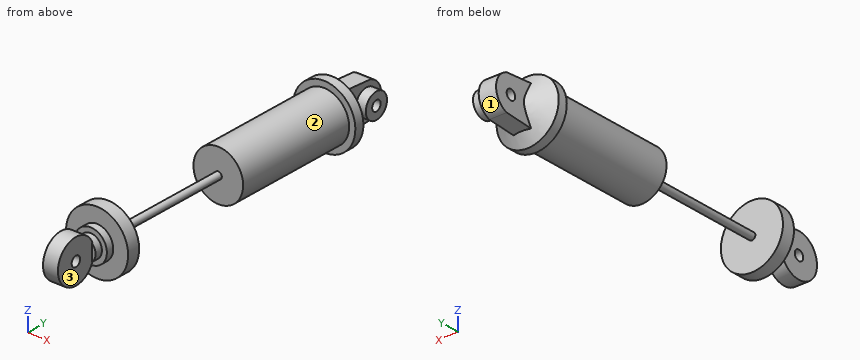
from build123d import *

# Parameters (mm, degrees)
SKETCH1_R      = 7.9375
EXTRUDE1_DEPTH = 70.485
SKETCH4_R      = 1.27
EXTRUDE2_DEPTH = 2.2225
SKETCH5_R      = 5.3975
SKETCH5_R_2    = 1.27
EXTRUDE3_DEPTH = 1.905
SKETCH6_R      = 4.1275
EXTRUDE4_DEPTH = 1.905
SKETCH7_R      = 2.8575
EXTRUDE5_DEPTH = 1.905
SKETCH8_R      = 3.175
SKETCH8_R_2    = 1.27
EXTRUDE6_DEPTH = 2.54
SKETCH9_R      = 7.9375
SKETCH9_R_2    = 6.35
EXTRUDE7_DEPTH = 33.02
SKETCH10_R     = 8.451029387
SKETCH10_R_2   = 0.889
EXTRUDE8_DEPTH = 33.02


with BuildPart() as part:
    # Sketch1 → Extrude1 (new body)
    with BuildSketch(Plane(origin=(0, 0, 0), x_dir=(1, 0, 0), z_dir=(0, 1, 0))):
        with Locations(Location((0, 0, 0), (0, 0, 270))):
            Circle(SKETCH1_R)
    extrude(amount=-EXTRUDE1_DEPTH)

    # Loft1: read off the stored shape, not the designer's step
    # Loft1: loft between two sections, ruled curve by curve
    loft1_from = [
        Edge.make_bspline([(3.207196431, 0, 7.26070226), (17.72860095, 0, 0.846309398), (11.314208088, 0, -13.675095122), (-3.207196431, 0, -7.26070226), (-17.72860095, 0, -0.846309398), (-11.314208088, 0, 13.675095122), (3.207196431, 0, 7.26070226)], [0, 0, 0, 0, 0.5, 0.5, 0.5, 1, 1, 1, 1], 3, [1, 0.333333333, 0.333333333, 1, 0.333333333, 0.333333333, 1]),
    ]
    loft1_to = [
        Edge.make_bspline([(0.075387957, 3.937, 1.903507724), (3.882403406, 3.937, 1.75273181), (3.731627491, 3.937, -2.054283639), (-0.075387957, 3.937, -1.903507724), (-3.882403406, 3.937, -1.75273181), (-3.731627491, 3.937, 2.054283639), (0.075387957, 3.937, 1.903507724)], [0, 0, 0, 0, 0.5, 0.5, 0.5, 1, 1, 1, 1], 3, [1, 0.333333333, 0.333333333, 1, 0.333333333, 0.333333333, 1]),
    ]
    loft1 = Solid(Shell([*[Face.make_surface_from_curves(loft1_from[k], loft1_to[k]) for k in range(1)], Face(Wire(loft1_from)), Face(Wire(loft1_to))]))
    add(loft1)

    # Sketch4 → Extrude2 (add, symmetric)
    with BuildSketch(Plane(origin=(0, 0, 0), x_dir=(0, 0, -1), z_dir=(1, 0, 0))):
        with BuildLine():
            Line((4.965601833, 1.905), (4.445, 8.89))
            ThreePointArc((4.445, 8.89), (0, 12.065), (-4.445, 8.89))
            Line((-4.445, 8.89), (-4.965601949, 1.905))
            Line((-4.965601949, 1.905), (-5.107584298, 0))
            Line((-5.107584298, 0), (5.107584151, 0))
            Line((5.107584151, 0), (4.965601833, 1.905))
        make_face()
        with Locations((0, 7.62)):
            Circle(SKETCH4_R, mode=Mode.SUBTRACT)
    extrude(amount=EXTRUDE2_DEPTH, both=True)

    # Sketch6 → Extrude4 (add)
    with BuildSketch(Plane.XZ.offset(70.485)):
        with Locations(Location((0, 0, 0), (0, 0, 90))):
            Circle(SKETCH6_R)
    extrude(amount=EXTRUDE4_DEPTH)



with BuildPart() as body_2:
    # Sketch5 → Extrude3 (new, symmetric)
    with BuildSketch(Plane(origin=(0, 0, 0), x_dir=(0, 0, -1), z_dir=(1, 0, 0))):
        with Locations(Location((0, -79.0575, 0), (0, 0, 180))):
            Circle(SKETCH5_R)
        with Locations(Location((0, -79.0575, 0), (0, 0, 180))):
            Circle(SKETCH5_R_2, mode=Mode.SUBTRACT)
    extrude(amount=EXTRUDE3_DEPTH, both=True)


with BuildPart() as part_1:
    add(part.part)

    add(body_2.part)  # Extrude5 merges body 2
    # Sketch7 → Extrude5 (add)
    with BuildSketch(Plane.XZ.offset(72.39)):
        with Locations(Location((0, 0, 0), (0, 0, 117.266044451))):
            Circle(SKETCH7_R)
    extrude(amount=EXTRUDE5_DEPTH)

    # Sketch8 → Extrude6 (add)
    with BuildSketch(Plane(origin=(2.2225, 0, 0), x_dir=(0, 0, -1), z_dir=(1, 0, 0))):
        with Locations(Location((0, 7.62, 0), (0, 0, 180))):
            Circle(SKETCH8_R)
        with Locations((0, 7.62)):
            Circle(SKETCH8_R_2, mode=Mode.SUBTRACT)
    extrude(amount=EXTRUDE6_DEPTH)

    # Sketch9 → Extrude7 (cut)
    with BuildSketch(Plane(origin=(0, -2.413, 0), x_dir=(-1, 0, 0), z_dir=(0, 1, 0))):
        with Locations(Location((0, 0, 0), (0, 0, 90))):
            Circle(SKETCH9_R)
        with Locations(Location((0, 0, 0), (0, 0, 90))):
            Circle(SKETCH9_R_2, mode=Mode.SUBTRACT)
    extrude(amount=-EXTRUDE7_DEPTH, mode=Mode.SUBTRACT)

    # Sketch10 → Extrude8 (cut)
    with BuildSketch(Plane(origin=(0, -34.163, 0), x_dir=(-1, 0, 0), z_dir=(0, 1, 0))):
        Circle(SKETCH10_R)
        with Locations(Location((0, 0, 0), (0, 0, 90))):
            Circle(SKETCH10_R_2, mode=Mode.SUBTRACT)
    extrude(amount=-EXTRUDE8_DEPTH, mode=Mode.SUBTRACT)


solid = part_1.part
Check sheet for the modelled part. Datum: model origin and axes. Units: mm. Face numbers are marked on the shaded views. Give positions to 0.01 mm unless a question says otherwise; leave off trailing zeros. Order: outer loops, then holes, each group sorted by start corner. A loop starts at its lowest first (then second) coordinate and runs counter-clockwise, first axis right, second up. Notation, with made-up numbers: (-8, -14) - (29, -14) arc R19 cw to (29, 16) - close; hole circle Ø2 at (-24.75, -37). An arc over 180 degrees is marked (long way). Answer as CSV lines item,"result".
1. Scan lines: probe 1 along Y at (x, z) = (3, 1); probe 2 along Y at (x, z) = (-2, -1) (3 decimals); probe 3 along Y at (x, z) = (1.5, -0.5). Record each from-to range of solid material in increasing order. Write a range as from..to.
Result sheet:
probe 1,"-72.39..-67.18, -34.16..3.08, 4.61..6.84, 8.4..10.63"
probe 2,"-74.295..-67.183, -34.163..6.837, 8.403..11.957"
probe 3,"-84.43..-80.22, -77.89..-67.18, -34.16..6.45, 8.79..12.04"
2. Section check D-D (y = -75.5). Record the boundary of the cut face in (x, z) (3 decimals).
Result sheet:
outline,"(-1.905, -4.059) - (1.905, -4.059) - (1.905, 4.059) - (-1.905, 4.059) - close"
3. Section check B-B (z = 0). State how many separate pieces and enclosed holes the cut face has, then the cut area to 3 significant figures.
Result sheet:
separate pieces,"3"
enclosed holes,"0"
area,"681 mm²"
4. Mould release check, pull along Y, two halves, no side actions. Record for the marked faces 1, 2 and 3: released by +Y, released by -Y, zero draft, split by the parting line, or undercut.
Result sheet:
face 1,"released by +Y"
face 2,"undercut"
face 3,"zero draft"
5. Section check A-A (y = 7.62). Record the boundary of the cut face in (x, z) (1 decimal), then the cut area to 3 significant figures.
Result sheet:
outline,"(-2.2, -4.5) - (2.2, -4.5) - (2.2, -3.2) - (4.8, -3.2) - (4.8, -1.3) - (-2.2, -1.3) - close; (-2.2, 1.3) - (4.8, 1.3) - (4.8, 3.2) - (2.2, 3.2) - (2.2, 4.5) - (-2.2, 4.5) - close"
area,"38.7 mm²"
6. Section check C-C (y = -43.5). Record the boundary of the cut face in (x, z).
Result sheet:
outline,"circle Ø1.78 at (0, 0)"
7. Go/stop test with flat-tipped pins: P1, Ø3, axis at y = 4.5, z = -1, coming from the +X side; P2, Ø6, axis at x = -3.5, y = -56, coming from the -Z side; P3, Ø5, axis at y = -79.5, z = -2.5, coming from the -X side (3 decimals); P4, Ø3, axis at x = -3, y = -46, coming from the +Z side. Record where each tip stops, or that it passes through.
Result sheet:
P1,"x = 4.76"
P2,"z = -0.74"
P3,"x = -1.905"
P4,"through"
